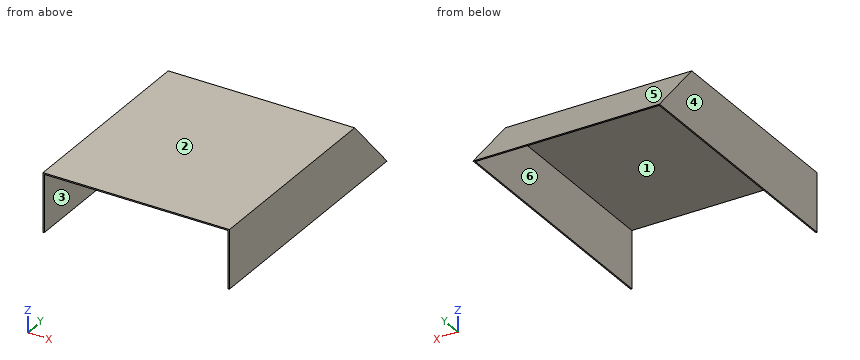
from build123d import *

# Parameters (mm, degrees)
F0_W     = 283
F0_H     = 390
F1_DEPTH = 88.9
F3_DEPTH = 283.001
F4_W     = 279
F4_H     = 86.9
F5_DEPTH = 390.001
F6_DEPTH = 281


with BuildPart() as f1:
    # F0 (on Top) → F1 (new body)
    with BuildSketch(Plane.XY):
        Rectangle(F0_W, F0_H)
    extrude(amount=F1_DEPTH)

    # F2 (on face) → F3 (cut, through all)
    with BuildSketch(Plane(origin=(-141.5, 0, 0), x_dir=(0, -1, 0), z_dir=(-1, 0, 0))):
        Polygon((-115, 88.9), (-195, 88.9), (-195, 0), align=None)
    extrude(amount=-F3_DEPTH, mode=Mode.SUBTRACT)

    # F4 (on face) → F5 (cut, through all)
    with BuildSketch(Plane.XZ.offset(195)):
        with Locations((0, 43.45)):
            Rectangle(F4_W, F4_H)
    extrude(amount=-F5_DEPTH, mode=Mode.SUBTRACT)

    # F2 (on face) → F6 (join, through all)
    with BuildSketch(Plane(origin=(-141.5, 0, 0), x_dir=(0, -1, 0), z_dir=(-1, 0, 0))):
        Polygon((-112.309426, 88.9), (-115, 88.9), (-195, 0), (-192.309426, 0), align=None)
    extrude(amount=-F6_DEPTH)


solid = f1.part
The listing builds one solid part. Answer for the finished solid, in the listing's coordinates (mm). Face numbers are marked on the shaded views. A direction names the side the tool comes from. Coordinates: 2 decimals unless noted, no trailing zeros. Loops run counter-clockwise (first coordinate to the right, second up) from the corner with the lowest first, then second, coordinate; pieces in that order, holes last. Notation, with made-up numbers: (-23, 81.5) -> (9, 81.5) arc R15 ccw to (9, 100.5) -> close; hole circle Ø3 at (21, 52). An arc over 180 degrees is marked (long way). Answer in a Markdown table with one row per item. Add a question column.
1. The part is cut by section C-C, the plane y = -136.5. Write down the section's boundary in (x, z).
2. Flat-ended cylindrical pins translate along their axes: P1, Ø6, axis at x = -58.5, z = 62.5, coming from the +Y side; P2, Ø6, axis at x = -61, z = 49, coming from the -Y side; P3, Ø12, axis at x = 28.5, y = -112.5, coming from the -Z side. Find the tip coordinate at first contact, or state that the pin passes through.
3. Determine the mould class of the marked faces 3, 4, 5 and 6 for opening direction X: +X half, -X half, draft (parallel to the pull), parting line (faces both ways), or undercut.
4. The part is cut by section A-A, the plane x = 124. Write down the section's boundary in (y, z).
5. The part is cut by section B-B, the plane z = 27. Write down the section's boundary in (x, y).
6. Consider line 1 (X direction, y = -72, z = 20.5); line 2 (Z direction, x = 95, y = 48.5); line 3 (Y direction, x = -88.5, z = 83). Determine where each line is inside the solid, lowest interval first. Write a range as [from, to].
7. For the marked faces 1 and 2, determine the directions among +Z, -Z, +X, -X, +Y, -Y from which every point of the face is accessible in a straight line to the end or side of a thin tool.
Answer below:
| question | item | result |
|---|---|---|
| 1 | outline | (-141.5, 0) -> (-139.5, 0) -> (-139.5, 86.9) -> (139.5, 86.9) -> (139.5, 0) -> (141.5, 0) -> (141.5, 88.9) -> (-141.5, 88.9) -> close |
| 2 | P1 | y = 141.46 |
| 2 | P2 | y = 145.52 |
| 2 | P3 | z = 86.9 |
| 3 | face 3 | undercut |
| 3 | face 4 | -X half |
| 3 | face 5 | draft |
| 3 | face 6 | undercut |
| 4 | outline | (-195, 86.9) -> (114.11, 86.9) -> (192.31, 0) -> (195, 0) -> (115, 88.9) -> (-195, 88.9) -> close |
| 5 | outline | (-141.5, -195) -> (-139.5, -195) -> (-139.5, 168.01) -> (139.5, 168.01) -> (139.5, -195) -> (141.5, -195) -> (141.5, 170.7) -> (-141.5, 170.7) -> close |
| 6 | line 1 | [-141.5, -139.5], [139.5, 141.5] |
| 6 | line 2 | [86.9, 88.9] |
| 6 | line 3 | [117.62, 120.31] |
| 7 | face 1 | -Z, -Y |
| 7 | face 2 | +Z, +X, -X, +Y, -Y |
